Design review of the part built by this model. Coordinates are the model's own, in mm. Face numbers are marked on the shaded views. A direction names the side the tool comes from. Give positions to 0.01 mm unless a question says otherwise; leave off trailing zeros. Loops run counter-clockwise (first coordinate to the right, second up) from the corner with the lowest first, then second, coordinate; pieces in that order, holes last. Notation, with made-up numbers: (76, 71.25) -> (129, 71.25) arc R12 cw to (129, 82.25) -> close; hole circle Ø5 at (-4.75, -26). An arc over 180 degrees is marked (long way). Use CSV: the item, a comma, the result in double quotes. Start each with the question number.
Item 1: We need section A-A (z = 0). State the section outline as (x, y) points.
Item 2: We need section B-B (y = 1). State the section outline as (x, z) points, plus the area to 3 significant figures.
Item 3: Wall thickness on line 1 along X through (y, z) = (6.75, -0.25); line 2 along Y through (x, z) = (8.25, -8.75); line 3 along X through (y, z) = (1.65, 11): over which ranges is each line inside the solid? List them lowest first. Write a range as from..to.
Item 4: The part is to be moulded in two halves that separate along Z. For the marked faces 3, 4, 5 and 6, say which applies: +Z half, -Z half, draft (parallel to the pull), parting line (faces both ways), or undercut.
Item 5: For the marked faces 1 and 2, list the 3-axis set-ups (+Z, -Z, +X, -X, +Y, -Y) from which the entire face can be reached by the end or side of a thin tool; tool diameter is ignored.
Item 6: We need section D-D (x = 0). Count the separate pieces of the cut face and the enclosed holes in it, plus the area to 3 significant figures.
Item 7: Clearance check with flat-ended pins moving along their axes: pin 1 (5.5 mm diameter, centred on x = 0, z = -11, fed in from -Y); pin 2 (1 mm diameter, centred on x = -2, z = -11, fed in from -Y); pin 3 (3 mm diameter, centred on x = 1, z = 1.5, fed in from +Y). State where each tip first meets the part, or that it passes through.
Item 8: We need section C-C (y = 6). State the section outline as (x, z) points, plus the area to 3 significant figures.
from build123d import *

# Parameters (mm, degrees)
SKETCH_1_R          = 15
EXTRUDE_1_DEPTH     = 2
SKETCH_2_R          = 7
EXTRUDE_2_DEPTH     = 8
SKETCH_3_R          = 5
CUT_EXTRUDE_1_DEPTH = 6
SKETCH_4_R          = 3
CUT_EXTRUDE_2_DEPTH = 23.045407685
CHAMFER_1_SIZE      = 0.5


with BuildPart() as part:
    # 草图1 → 凸台-拉伸1 (new body)
    with BuildSketch(Plane(origin=(0, 0, 0), x_dir=(1, 0, 0), z_dir=(0, 1, 0))):
        with Locations(Location((0, 0, 0), (0, 0, 270))):
            Circle(SKETCH_1_R)
    extrude(amount=EXTRUDE_1_DEPTH)

    # 草图2 → 凸台-拉伸2 (add)
    with BuildSketch(Plane(origin=(0, 2, 0), x_dir=(1, 0, 0), z_dir=(0, 1, 0))):
        with Locations(Location((0, 0, 0), (0, 0, 270))):
            Circle(SKETCH_2_R)
    extrude(amount=EXTRUDE_2_DEPTH)

    # 草图3 → 切除-拉伸1 (cut)
    with BuildSketch(Plane(origin=(0, 10, 0), x_dir=(1, 0, 0), z_dir=(0, 1, 0))):
        with Locations(Location((0, 0, 0), (0, 0, 270))):
            Circle(SKETCH_3_R)
    extrude(amount=-CUT_EXTRUDE_1_DEPTH, mode=Mode.SUBTRACT)

    # 草图4 → 切除-拉伸2 (cut, through all)
    with BuildSketch(Plane(origin=(0, 4, 0), x_dir=(1, 0, 0), z_dir=(0, 1, 0))):
        with Locations(Location((0, 0, 0), (0, 0, 270))):
            Circle(SKETCH_4_R)
    extrude(amount=-CUT_EXTRUDE_2_DEPTH, mode=Mode.SUBTRACT)

    # 倒角1
    chamfer_1_edges = [part.edges().sort_by_distance(p)[0] for p in [
        (0, 10, -5),
        (0, 0, -3),
        (0, 0, -15),
        (0, 10, -7),
    ]]
    chamfer(chamfer_1_edges, length=CHAMFER_1_SIZE)

    # 草图8 → M6 内六角花形半沉头螺钉的锥形沉头孔1 (revolve, cut)
    with BuildSketch(Plane(origin=(0, 0, 11), x_dir=(0, 0, -1), z_dir=(1, 0, 0))):
        Polygon((0, 0), (0, 3.65), (1.65, 2), (1.65, 1.35), (3, 0), align=None)
    hole_wizard_m6_1 = revolve(axis=Axis((0, -6.35, 11), (0, 1, 0)), mode=Mode.SUBTRACT)

    # 镜向1: M6 内六角花形半沉头螺钉的锥形沉头孔1 across plane
    add(hole_wizard_m6_1.mirror(Plane.XY), mode=Mode.SUBTRACT)


solid = part.part
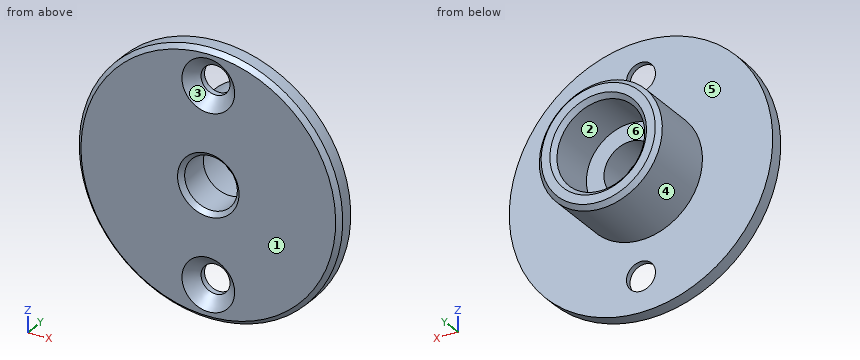
Results found:
1,outline,"(-15, 0.5) -> (-14.5, 0) -> (-3.5, 0) -> (-3, 0.5) -> (-3, 4) -> (-5, 4) -> (-5, 9.5) -> (-5.5, 10) -> (-6.5, 10) -> (-7, 9.5) -> (-7, 2) -> (-15, 2) -> close; (3, 0.5) -> (3.5, 0) -> (14.5, 0) -> (15, 0.5) -> (15, 2) -> (7, 2) -> (7, 9.5) -> (6.5, 10) -> (5.5, 10) -> (5, 9.5) -> (5, 4) -> (3, 4) -> close"
2,outline,"circle Ø30 at (0, 0); hole circle Ø6 at (0, 0); hole circle Ø4 at (0, -11); hole circle Ø4 at (0, 11)"
2,area,"653 mm²"
3,line 1,"-7..-4.99, 4.99..7"
3,line 2,"0..2"
3,line 3,"-10.2..-1.65, 1.65..10.2"
4,face 3,"undercut"
4,face 4,"parting line"
4,face 5,"draft"
4,face 6,"undercut"
5,face 1,"+Z, -Z, +X, -X, -Y"
5,face 2,"+Y"
6,separate pieces,"4"
6,enclosed holes,"0"
6,area,"70.2 mm²"
7,pin 1,"y = 0.25"
7,pin 2,"y = 0.5"
7,pin 3,"y = 4"
8,outline,"circle Ø14 at (0, 0); hole circle Ø10 at (0, 0)"
8,area,"75.4 mm²"
